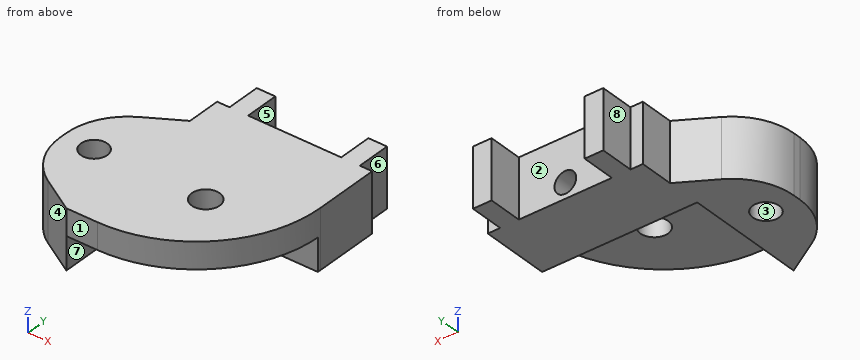
Autodesk Inventor part; units mm, degrees
ref_plane "YZ Plane" through (0, 0, 0) normal (1, 0, 0) x (0, 1, 0)
ref_plane "XZ Plane" through (0, 0, 0) normal (0, 1, 0) x (-1, 0, 0)
ref_plane "XY Plane" through (0, 0, 0) normal (0, 0, 1) x (1, 0, 0)
sketch "Sketch1" plane through (0, 0, 0) normal (0, 0, 1) x (1, 0, 0)
  line L0 (-21, -21) -> (21, -21)
  line L1 (21, -21) -> (21, 21)
  line L2 (21, 21) -> (-21, 21)
  line L3 (-21, 21) -> (-21, -21)
  line L4 (-21, -21) -> (21, 21) construction
  line L5 (21, -21) -> (-21, 21) construction
  circle A0 centre (0, 0) radius 4.5
  circle A1 centre (-36, 0) radius 4.25
  line L6 (-46, 0) -> (-46, 12.5)
  line L7 (-46, 0) -> (-46, -12.5)
  line L8 (-25, -25) -> (25, -25)
  line L9 (25, -25) -> (25, 25)
  line L10 (-25, -25) -> (25, 25) construction
  line L11 (25, -25) -> (-25, 25) construction
  line L12 (-46, 12.5) -> (-25, 25)
  line L13 (-46, -12.5) -> (-25, -25)
  line L14 (0, 36) -> (15, 36)
  line L15 (15, 36) -> (15, 47)
  line L16 (15, 47) -> (21, 47)
  line L17 (21, 47) -> (21, 36)
  line L18 (21, 36) -> (25, 36)
  line L19 (25, 36) -> (25, 25)
  line L20 (0, 36) -> (-15, 36)
  line L21 (-15, 36) -> (-15, 47)
  line L22 (-15, 47) -> (-21, 47)
  line L23 (-21, 47) -> (-21, 36)
  line L24 (-21, 36) -> (-25, 36)
  line L25 (-25, 36) -> (-25, 25)
  line L26 (-25, 25) -> (25, 25)
  dimension "d0" = 42
  dimension "d1" = 42
  dimension "d2" = 9
  dimension "d5" = 8.5
  dimension "d6" = 46
  dimension "d10" = 50
  dimension "d12" = 15
  dimension "d14" = 6
  dimension "d15" = 11
  dimension "d21" = 11
  dimension "d22" = 50
  dimension "d23" = 25
  dimension "d24" = 4
extrude "Extrusion1" add sketch "Sketch1" along normal blind 15 contours L3 L2 L1 L0 | L6 L12 L26 L9 L8 L13 L7 | L25 L24 L23 L22 L21 L20 L14 L15 L16 L17 L18 L19 L26
move faces "Move1" translate (0, 0, 10) faces at (0.1808, -18.1557, 15)
sketch "Sketch2" plane through (-25, -25, 25) normal (0, 0, 1) x (1, 0, 0)
  line L0 (0, 5) -> (50, 45) construction
  line L1 (50, 5) -> (0, 45) construction
  line L2 (50, 0) -> (50, 61)
  line L3 (50, 0) -> (0, 0)
  line L4 (0, 0) -> (0, 40)
  line L5 (0, 40) -> (50, 40)
  line L6 (50, 40) -> (50, 0)
  point P0 (25, 25)
  dimension "d32" = 50
  dimension "d33" = 40
sketch "Sketch3" plane through (-25, -25, 25) normal (0, 0, 1) x (1, 0, 0)
  line L0 (50, 0) -> (50, 61)
  line L1 (50, 0) -> (0, 0)
  line L2 (0, 0) -> (0, 38)
  line L3 (0, 38) -> (50, 38)
  line L4 (50, 38) -> (50, 0)
  point P0 (25, 25)
  dimension "d34" = 50
  dimension "d35" = 38
move faces "Move2" translate (0, 0, -2) faces at (18.1231, 4.0256, 25)
move faces "Move3" translate (0, 0, 4) faces at (18.1231, 4.0256, 0)
sketch "Sketch5" plane through (25, -25, 4) normal (0, 0, -1) x (-1, 0, 0)
  line L0 (0, 0) -> (0, 61)
  line L1 (0, 0) -> (50, 0)
  line L2 (50, 0) -> (50, 39)
  line L3 (50, 39) -> (0, 39)
  line L4 (0, 39) -> (0, 0)
  point P0 (25, 25)
  point P1 (0, 39)
  dimension "d48" = 50
  dimension "d49" = 39
extrude "Extrusion4" cut sketch "Sketch5" against normal blind 10
sketch "Sketch6" plane through (-25, 14, 4) normal (0, -1, 0) x (1, 0, 0)
  circle A0 centre (25, 5) radius 3.5
  line L0 (50, 0) -> (0, 0)
  point P0 (25, -4)
  dimension "d52" = 7
  dimension "d53" = 5
move faces "Move4" translate (0, 0, 0.5) faces at (0.1808, -18.1557, 14)
extrude "Extrusion5" cut sketch "Sketch6" against normal blind 30
fillet "Fillet1" radius 40 1 edges at (25, -25, 18.75)
fillet "Fillet2" radius 20 1 edges at (-46, -12.5, 13.5)
fillet "Fillet3" radius 20 1 edges at (-46, 12.5, 13.5)
properties part number "SuporteInferior"
Source: CAD feature listing. Evaluate the final solid. Frame: model axes, mm. Face numbers are marked on the shaded views. A direction names the side the tool comes from. Give positions to 0.01 mm unless a question says otherwise; leave off trailing zeros. Write each loop counter-clockwise with the first axis right and the second up, starting at its lowest first coordinate (ties: lowest second). Pieces come first, ordered by that corner, then holes. Notation, with made-up numbers: (-20, 22.5) - (16, 22.5) arc R22 ccw to (16, 51.5) - close; hole circle Ø4 at (49.25, 15.25). An arc over 180 degrees is marked (long way). One line per item, written item: value. Start each with the question number.
Q1. Draft query along X for the marked faces 1, 2, 3 and 4. Return one class per face: +X half, -X half, draft (parallel to the pull), parting line (faces both ways), or undercut.
Q2. Section query B-B, the plane x = 0. Return the cut outline in (y, z).
Q3. Material intervals for probe 1 along Z at (x, y) = (0, 24.5); probe 2 along X at (y, z) = (0, 8); probe 3 along Z at (x, y) = (-8, -17.5), sorted ascending. Write a range as from..to.
Q4. First-contact query: pin 1 Ø5 at (x, z) = (0, 9.5) entering from -Y; pin 2 Ø1.5 at (y, z) = (-9, 9.5) entering from +X; pin 3 Ø5.5 at (y, z) = (43.5, 17.5) entering from +X; pin 4 Ø9.5 at (x, z) = (-2.5, 13) entering from +Y. Flat tips, straight axial feed; report the tip coordinate or a pass-through.
Q5. Section query C-C, the plane y = 0. Return the cut outline in (x, z).
Q6. Section query D-D, the plane z = 17.25. Return the cut outline in (x, y).
Q7. Section query A-A, the plane z = 9. Return the cut outline in (x, y).
Q8. Set-up query: the marked faces 5, 6, 7 and 8. Return all of +Z, -Z, +X, -X, +Y, -Y with unobstructed straight access to the full face (end or side cutting, diameter ignored); none if empty.
Answer:
1. face 1: draft
1. face 2: undercut
1. face 3: undercut
1. face 4: -X half
2. outline: (-22.08, 14.5) - (-4.5, 14.5) - (-4.5, 23) - (-22.08, 23) - close; (4.5, 14.5) - (14, 14.5) - (14, 12.5) - (36, 12.5) - (36, 23) - (4.5, 23) - close; (14, 4) - (36, 4) - (36, 5.5) - (14, 5.5) - close
3. probe 1: z = 4..5.5, 12.5..23
3. probe 2: x = -46..-40.25, -31.75..-25
3. probe 3: z = 14.5..23
4. pin 1: passes through
4. pin 2: stops at x = -25
4. pin 3: stops at x = 21
4. pin 4: stops at y = 36
5. outline: (-46, 4) - (-40.25, 4) - (-40.25, 23) - (-46, 23) - close; (-31.75, 4) - (-25, 4) - (-25, 14.5) - (-4.5, 14.5) - (-4.5, 23) - (-31.75, 23) - close; (4.5, 14.5) - (22.08, 14.5) - (22.08, 23) - (4.5, 23) - close
6. outline: (-46, -1.13) arc R20 ccw to (-36.23, -18.32) - (-25, -25) - (-15, -25) arc R40 ccw to (25, 15) - (25, 36) - (21, 36) - (21, 47) - (15, 47) - (15, 36) - (-15, 36) - (-15, 47) - (-21, 47) - (-21, 36) - (-25, 36) - (-25, 25) - (-36.23, 18.32) arc R20 ccw to (-46, 1.13) - close; hole circle Ø8.5 at (-36, 0); hole circle Ø9 at (0, 0)
7. outline: (-46, -1.13) arc R20 ccw to (-36.23, -18.32) - (-25, -25) - (-25, 14) - (-3.5, 14) - (-3.5, 36) - (-15, 36) - (-15, 47) - (-21, 47) - (-21, 36) - (-25, 36) - (-25, 25) - (-36.23, 18.32) arc R20 ccw to (-46, 1.13) - close; (3.5, 14) - (24.99, 14) arc R40 ccw to (25, 15) - (25, 36) - (21, 36) - (21, 47) - (15, 47) - (15, 36) - (3.5, 36) - close; hole circle Ø8.5 at (-36, 0)
8. face 5: +Z, -Z, +Y
8. face 6: +Z, -Z, +X, +Y
8. face 7: -Z, +X, -Y
8. face 8: +Z, -Z, -X, +Y
